The listing builds one solid part. Answer for the finished solid, in the listing's coordinates (mm). A direction names the side the tool comes from. Coordinates: 2 decimals unless noted, no trailing zeros. Loops run counter-clockwise (first coordinate to the right, second up) from the corner with the lowest first, then second, coordinate; pieces in that order, holes last. Notation, with made-up numbers: (-10, 29) - (32, 29) arc R26 ccw to (32, 45) - close; hole circle Ø7 at (-6, -12.5). An arc over 180 degrees is marked (long way). Return JSON: item names as keys, results as strings. Group by question number.
1. Section D-D (y = 97) is taken. Write down the section's boundary in (x, z).
2. Which of the six approach directions +Z, -Z, +X, -X, +Y, -Y give full straight-line access (tool end or side, diameter ignored) to faces 1 (the face through (25.4, 394, -13)), 2 (the face through (452, 355.6, 26)), 3 (the face through (902, 25.4, -13)), 4 (the face through (452, 203, 0))?
3. The mould has two halves that part along Y. Classify faces 5 (the face through (13, 394, -25.4)), 6 (the face through (451, 406.4, 22)), 7 (the face through (25, 153, 0)): pulls with the +Y half, pulls with the -Y half, needs draft (parallel to the pull), parting line crosses it, or undercut.
4. Find the intervals of material crossed by line 1 along Y through (x, z) = (619, -3); line 2 along Y through (x, z) = (532.5, 0.5); line 3 along X through (y, z) = (83, 5.5), in increasing order.
5. Section B-B (z = 18) is taken. Write down the section's boundary in (x, y), and give its area (3 significant figures).
6. Section C-C (y = 266) is taken. Write down the section's boundary in (x, z), and give its area (3 significant figures).
7. Each of these flat-tipped pins is pushed along its axis until it touches: P1, Ø7.5, axis at x = 352.5, z = -17, coming from the -Y side; P2, Ø5, axis at x = 290.5, y = 211, coming from the +Z side; P3, Ø7.5, axis at x = 489, z = -19, coming from the +Y side. Where does it stop, or does it pass through?
8. Section A-A (x = 357) is taken. Write down the section's boundary in (y, z).
```python
from build123d import *

# Parameters (mm, degrees)
SKETCH_W     = 914.4
SKETCH_H     = 406.4
PAD_DEPTH    = 50.8
SKETCH001_W  = 812.8
SKETCH001_H  = 304.8
POCKET_DEPTH = 50.801
SKETCH002_W  = 914.4
SKETCH002_H  = 50.8
PAD001_DEPTH = 25.4
SKETCH003_W  = 25.4
SKETCH003_H  = 25.4
PAD002_DEPTH = 25.4


with BuildPart() as part:
    # Sketch → Pad (new body)
    with BuildSketch(Plane.XY):
        with Locations((457.2, 203.2)):
            Rectangle(SKETCH_W, SKETCH_H)
    extrude(amount=PAD_DEPTH)

    # Sketch001 (on Face6 of Pad) → Pocket (cut, through all)
    with BuildSketch(Plane.XY.offset(50.8)):
        with Locations((457.2, 203.2)):
            Rectangle(SKETCH001_W, SKETCH001_H)
    extrude(amount=-POCKET_DEPTH, mode=Mode.SUBTRACT)

    # Sketch002 (on Face4 of Pocket) → Pad001 (join)
    with BuildSketch(Plane(origin=(0, 0, 0), x_dir=(1, 0, 0), z_dir=(0, 0, -1))):
        with Locations((457.2, -101.6)):
            Rectangle(SKETCH002_W, SKETCH002_H)
        with Locations((457.2, -203.2)):
            Rectangle(SKETCH002_W, SKETCH002_H)
        with Locations((457.2, -304.8)):
            Rectangle(SKETCH002_W, SKETCH002_H)
    extrude(amount=PAD001_DEPTH)

    # Sketch003 (on Face4 of Pad001) → Pad002 (join)
    with BuildSketch(Plane(origin=(0, 0, 0), x_dir=(1, 0, 0), z_dir=(0, 0, -1))):
        with Locations((12.7, -393.7)):
            Rectangle(SKETCH003_W, SKETCH003_H)
        with Locations((901.7, -393.7)):
            Rectangle(SKETCH003_W, SKETCH003_H)
        with Locations((901.7, -12.7)):
            Rectangle(SKETCH003_W, SKETCH003_H)
        with Locations((12.7, -12.7)):
            Rectangle(SKETCH003_W, SKETCH003_H)
    extrude(amount=PAD002_DEPTH)


solid = part.part
```
The answers:
{
 "1": {"outline": "(0, -25.4) - (914.4, -25.4) - (914.4, 50.8) - (863.6, 50.8) - (863.6, 0) - (50.8, 0) - (50.8, 50.8) - (0, 50.8) - close"},
 "2": {"face 1": "-Z, +Y", "face 2": "+Z, -Z", "face 3": "-Z, +X, -X", "face 4": "+Z"},
 "3": {"face 5": "needs draft", "face 6": "pulls with the +Y half", "face 7": "undercut"},
 "4": {"line 1": "y = 76.2 to 127, 177.8 to 228.6, 279.4 to 330.2", "line 2": "y = 0 to 50.8, 355.6 to 406.4", "line 3": "x = 0 to 50.8, 863.6 to 914.4"},
 "5": {"outline": "(0, 0) - (914.4, 0) - (914.4, 406.4) - (0, 406.4) - close; hole (50.8, 50.8) - (863.6, 50.8) - (863.6, 355.6) - (50.8, 355.6) - close", "area": "124,000 mm2"},
 "6": {"outline": "(0, 0) - (50.8, 0) - (50.8, 50.8) - (0, 50.8) - close; (863.6, 0) - (914.4, 0) - (914.4, 50.8) - (863.6, 50.8) - close", "area": "5,160 mm2"},
 "7": {"P1": "stops at y = 76.2", "P2": "stops at z = 0", "P3": "stops at y = 330.2"},
 "8": {"outline": "(0, 0) - (50.8, 0) - (50.8, 50.8) - (0, 50.8) - close; (76.2, -25.4) - (127, -25.4) - (127, 0) - (76.2, 0) - close; (177.8, -25.4) - (228.6, -25.4) - (228.6, 0) - (177.8, 0) - close; (279.4, -25.4) - (330.2, -25.4) - (330.2, 0) - (279.4, 0) - close; (355.6, 0) - (406.4, 0) - (406.4, 50.8) - (355.6, 50.8) - close"}
}
